```python
from build123d import *

# Parameters (mm, degrees)
SKIZZE1_R                       = 9.165
AUFSATZ_LINEAR_AUSTRAGEN1_DEPTH = 3.063
SKIZZE20_R                      = 6.6
AUFSATZ_LINEAR_AUSTRAGEN4_DEPTH = 0.69
SKIZZE21_R                      = 6.6
AUFSATZ_LINEAR_AUSTRAGEN5_DEPTH = 1.3
SKIZZE22_R                      = 4
AUFSATZ_LINEAR_AUSTRAGEN6_DEPTH = 6.6
SKIZZE22_3_R                    = 4
AUFSATZ_LINEAR_AUSTRAGEN7_DEPTH = 5.98
SKIZZE28_R                      = 8.315
AUFSATZ_LINEAR_AUSTRAGEN8_DEPTH = 0.6
SKIZZE29_R                      = 5.435
AUFSATZ_LINEAR_AUSTRAGEN9_DEPTH = 36.75
VERRUNDUNG1_R                   = 0.6
FASE1_SIZE                      = 1.5


with BuildPart() as part:
    # Skizze1 → Aufsatz-Linear austragen1 (new body)
    with BuildSketch(Plane(origin=(0, 0, 0), x_dir=(1, 0, 0), z_dir=(0, 1, 0))):
        with Locations(Location((0, 0, 0), (0, 0, 270))):  # turned: the seam where the file's is
            Circle(SKIZZE1_R)
    extrude(amount=AUFSATZ_LINEAR_AUSTRAGEN1_DEPTH)

    # Skizze19 → Rotation1 (revolve)
    with BuildSketch(Plane.XY, mode=Mode.PRIVATE) as rotation1_sk:
        Polygon((6.6, 3.063), (6.6, 3.753), (9.165, 3.063), align=None)
    revolve(rotation1_sk.sketch.rotate(Axis((0, 0, 0), (0, 1, 0)), 90), axis=Axis((0, 0, 0), (0, 1, 0)))  # turned: the seam where the file's is

    # Skizze20 → Aufsatz-Linear austragen4 (add)
    with BuildSketch(Plane(origin=(0, 3.063, 0), x_dir=(1, 0, 0), z_dir=(0, 1, 0))):
        Circle(SKIZZE20_R)
    extrude(amount=AUFSATZ_LINEAR_AUSTRAGEN4_DEPTH)

    # Skizze21 → Aufsatz-Linear austragen5 (add)
    with BuildSketch(Plane(origin=(0, 3.753, 0), x_dir=(1, 0, 0), z_dir=(0, 1, 0))):
        with Locations(Location((0, 0, 0), (0, 0, 270))):  # turned: the seam where the file's is
            Circle(SKIZZE21_R)
    extrude(amount=AUFSATZ_LINEAR_AUSTRAGEN5_DEPTH)

    # Skizze22 → Aufsatz-Linear austragen6 (add)
    with BuildSketch(Plane(origin=(0, 5.053, 0), x_dir=(1, 0, 0), z_dir=(0, 1, 0))):
        with Locations(Location((0, 0, 0), (0, 0, 270))):  # turned: the seam where the file's is
            Circle(SKIZZE22_R)
    extrude(amount=AUFSATZ_LINEAR_AUSTRAGEN6_DEPTH)

    # Skizze22_3 → Aufsatz-Linear austragen7 (add)
    with BuildSketch(Plane(origin=(0, 5.053, 0), x_dir=(1, 0, 0), z_dir=(0, 1, 0))):
        with BuildLine():
            ThreePointArc((1, 5.325), (0, 6.325), (-1, 5.325))
            ThreePointArc((-1, 5.325), (-2.295031806, 3.971342442), (-4.115915402, 3.531025404))
            ThreePointArc((-4.115915402, 3.531025404), (-4.821728224, 3.643591377), (-5.42240304, 3.256250954))
            ThreePointArc((-5.42240304, 3.256250954), (-5.477610679, 3.1625), (-5.531197567, 3.067813305))
            ThreePointArc((-5.531197567, 3.067813305), (-5.566306805, 2.353943444), (-5.115915402, 1.798974596))
            ThreePointArc((-5.115915402, 1.798974596), (-4.588162786, 0), (-5.115915402, -1.798974596))
            ThreePointArc((-5.115915402, -1.798974596), (-5.566306805, -2.353943444), (-5.531197567, -3.067813305))
            ThreePointArc((-5.531197567, -3.067813305), (-5.477610679, -3.1625), (-5.42240304, -3.256250954))
            ThreePointArc((-5.42240304, -3.256250954), (-4.821728224, -3.643591377), (-4.115915402, -3.531025404))
            ThreePointArc((-4.115915402, -3.531025404), (-2.295031806, -3.971342442), (-1, -5.325))
            ThreePointArc((-1, -5.325), (0, -6.325), (1, -5.325))
            ThreePointArc((1, -5.325), (2.295031806, -3.971342442), (4.115915402, -3.531025404))
            ThreePointArc((4.115915402, -3.531025404), (5.477610679, -3.1625), (5.115915402, -1.798974596))
            ThreePointArc((5.115915402, -1.798974596), (4.586799345, -0.001884626), (5.111585275, 1.796474596))
            ThreePointArc((5.111585275, 1.796474596), (5.477610679, 3.1625), (4.111585275, 3.528525404))
            ThreePointArc((4.111585275, 3.528525404), (2.29239063, 3.970537041), (1, 5.325))
        make_face()
        with Locations(Location((0, 0, 0), (0, 0, 270))):  # turned: the seam where the file's is
            Circle(SKIZZE22_3_R, mode=Mode.SUBTRACT)
    extrude(amount=AUFSATZ_LINEAR_AUSTRAGEN7_DEPTH)

    # Skizze28 → Aufsatz-Linear austragen8 (add)
    with BuildSketch(Plane.XZ):
        with Locations(Location((0, 0, 0), (0, 0, 90))):  # turned: the seam where the file's is
            Circle(SKIZZE28_R)
    extrude(amount=AUFSATZ_LINEAR_AUSTRAGEN8_DEPTH)

    # Skizze29 → Aufsatz-Linear austragen9 (add)
    with BuildSketch(Plane.XZ.offset(0.6)):
        with Locations(Location((0, 0, 0), (0, 0, 270))):  # turned: the seam where the file's is
            Circle(SKIZZE29_R)
    extrude(amount=AUFSATZ_LINEAR_AUSTRAGEN9_DEPTH)

    # Verrundung1
    verrundung1_edges = [part.edges().sort_by_distance(p)[0] for p in [
        (0, -0.6, 5.435),
    ]]
    fillet(verrundung1_edges, radius=VERRUNDUNG1_R)

    # Skizze32 → Rotation3 (revolve)
    with BuildSketch(Plane.XY, mode=Mode.PRIVATE) as rotation3_sk:
        Polygon((4.611951316, 5.053), (4.611951316, 8.373), (6.6, 5.053), align=None)
    revolve(rotation3_sk.sketch.rotate(Axis((0, 0, 0), (0, 1, 0)), 270), axis=Axis((0, 0, 0), (0, 1, 0)))  # turned: the seam where the file's is

    # Fase1
    fase1_edges = [part.edges().sort_by_distance(p)[0] for p in [
        (0, -37.35, 5.435),
    ]]
    chamfer(fase1_edges, length=FASE1_SIZE)


solid = part.part
```
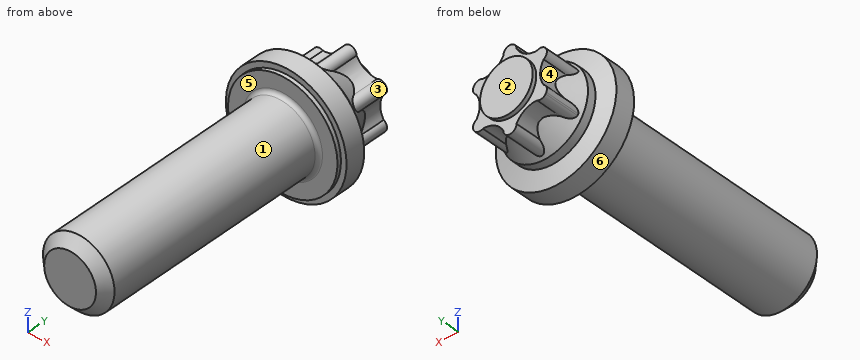
Geometry: final body of the model. Coordinates: model frame, mm. Face numbers are marked on the shaded views. A direction names the side the tool comes from. Round coordinates to 2 decimals unless told otherwise and drop trailing zeros. Order: outer loops, then holes, each group sorted by start corner. A loop starts at its lowest first (then second) coordinate and runs counter-clockwise, first axis right, second up. Notation, with made-up numbers: (64, 21) -> (103, 21) arc R14 ccw to (103, 34) -> close; hole circle Ø8 at (0.5, 15.5). An arc over 180 degrees is marked (long way). Use one line per item in the form item = value. Start each with the question number.
1. Cut plane B-B (x = 0). Return the cut outline in (y, z) (3 decimals).
2. Line query: probe 1 along Y at (x, z) = (-4.75, 5.75); probe 2 along Z at (x, y) = (7.25, 1); probe 3 along X at (y, z) = (-25.5, 2). Output: solid intervals per line, ascending.
3. Cut plane A-A (y = 6). Count the separate pieces of the cut face and the enclosed holes in it, then the cut area to 3 significant figures.
4. Cut plane C-C (y = -8). Return the cut outline in (x, z) (3 decimals), then the cut area to 3 significant figures.
5. Draft query along Z for the marked faces 3, 4, 5 and 6. Return one class per face: pulls with the +Z half, pulls with the -Z half, needs draft (parallel to the pull), parting line crosses it, or undercut.
6. Reachability of the marked faces 1 and 2 from +Z, -Z, +X, -X, +Y, -Y: full face, straight path, thin tool, end or side. Return the list, or none.
7. Pin query (flat end, axial travel): pin 1 Ø8 at (y, z) = (-11, 4) entering from +X (3 decimals); pin 2 Ø10 at (x, z) = (7, 1) entering from -Y; pin 3 Ø5 at (x, z) = (-5, 7) entering from -Y; pin 4 Ø5 at (y, z) = (-32.5, 4) entering from +X. Return the tip coordinate at first contact, or that it passes through.
Solution:
q1.outline = (-37.35, -3.935) -> (-35.85, -5.435) -> (-1.2, -5.435) arc R0.6 cw to (-0.6, -6.035) -> (-0.6, -8.315) -> (0, -8.315) -> (0, -9.165) -> (3.063, -9.165) -> (3.753, -6.6) -> (5.053, -6.6) -> (5.512, -6.325) -> (11.033, -6.325) -> (11.033, -4) -> (11.653, -4) -> (11.653, 4) -> (11.033, 4) -> (11.033, 6.325) -> (5.512, 6.325) -> (5.053, 6.6) -> (3.753, 6.6) -> (3.063, 9.165) -> (0, 9.165) -> (0, 8.315) -> (-0.6, 8.315) -> (-0.6, 6.035) arc R0.6 cw to (-1.2, 5.435) -> (-35.85, 5.435) -> (-37.35, 3.935) -> close
q2.probe_1 = -0.6 to 3.52
q2.probe_2 = -5.61 to 5.61
q2.probe_3 = -5.05 to 5.05
q3.separate_pieces = 1
q3.enclosed_holes = 6
q3.area = 116 mm^2
q4.outline = circle Ø10.87 at (0, 0)
q4.area = 92.8 mm^2
q5.face_3 = undercut
q5.face_4 = undercut
q5.face_5 = needs draft
q5.face_6 = parting line crosses it
q6.face_1 = -Y
q6.face_2 = +Z, -Z, +X, -X, +Y
q7.pin_1 = 5.435
q7.pin_2 = -37.35
q7.pin_3 = -0.6
q7.pin_4 = 5.22
